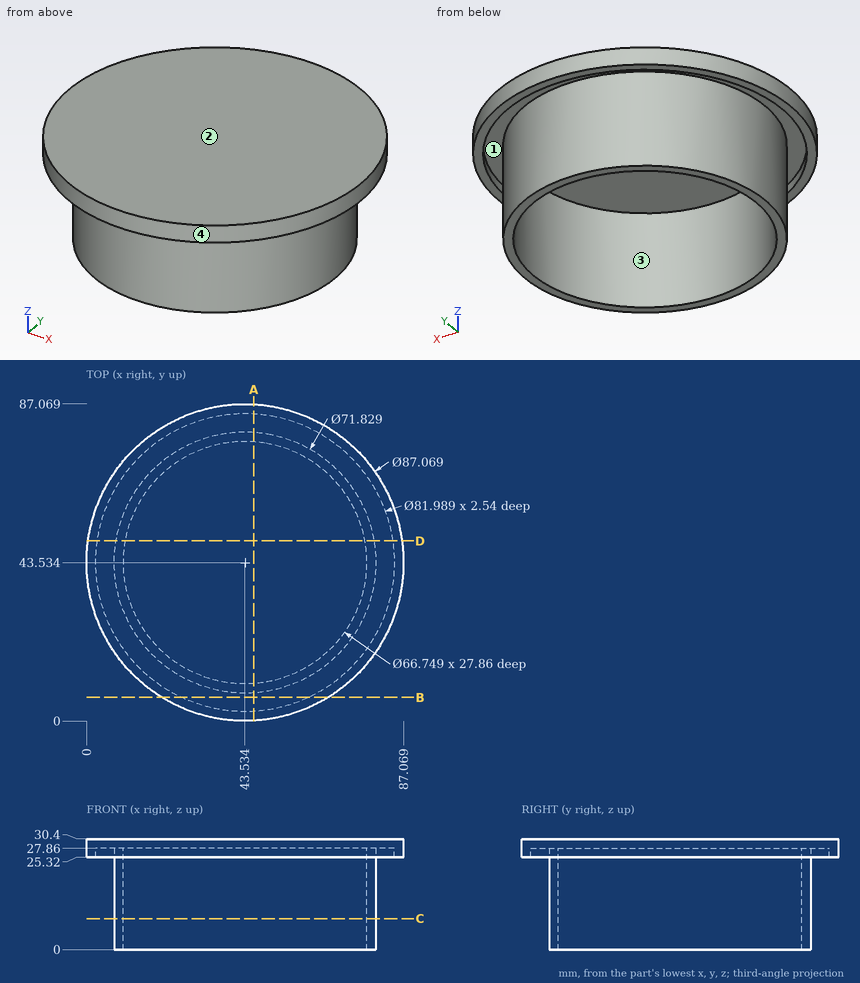
Source: three-view drawing plus pictorial views. Frame: mm from the lowest corner of the part. Coordinates: 2 decimals unless noted, no trailing zeros. Loops run counter-clockwise (first coordinate to the right, second up) from the corner with the lowest first, then second, coordinate; pieces in that order, holes last. Notation, with made-up numbers: (-26.75, 81) - (12.25, 81) arc R34 ccw to (12.25, 112) - close; hole circle Ø1 at (72, -22.75). An arc over 180 degrees is marked (long way). Answer in a Markdown table with one row per item. Add a question column.
Item 1: Contact query for flat-ended pins moving along their axis: P1, Ø1, axis at x = 64, z = 15.5, coming from the -Y side; P2, Ø6, axis at x = 51, y = 46.5, coming from the -Z side; P3, Ø1.5, axis at y = 56, z = 17, coming from the +X side (1 decimal). Output: stop coordinate, or through.
Item 2: Section query B-B on y = 6.5. Return the cut outline in (x, z), then the cut area to 3 significant figures.
Item 3: Section query C-C on z = 8.5. Return the cut outline in (x, y) (1 decimal).
Item 4: Section query A-A on x = 46. Return the cut outline in (y, z) (1 decimal).
Item 5: Mould query, pull axis X, two halves, no side actions, for the marked faces 1, 2, 3 and 4. Classes: released by +X, released by -X, zero draft, split by the parting line, or undercut.
Item 6: Line query: line 1 along Z through (x, y) = (21.5, 57.5); line 2 along X through (y, z) = (21, 24) (1 decimal); line 3 along Y through (x, z) = (32, 6.5) (1 decimal). Output: solid intervals per line, ascending. Write a range as [from, to].
Item 7: Section query D-D on y = 49.5. Return the cut outline in (x, z).
Recorded:
| question | item | result |
|---|---|---|
| 1 | P1 | y = 13.68 |
| 1 | P2 | z = 27.86 |
| 1 | P3 | x = 77.5 |
| 2 | outline | (20.65, 25.32) - (25.96, 25.32) - (25.96, 27.86) - (61.11, 27.86) - (61.11, 25.32) - (66.42, 25.32) - (66.42, 30.4) - (20.65, 30.4) - close |
| 2 | area | 143 mm^2 |
| 3 | outline | circle Ø71.8 at (43.5, 43.5); hole circle Ø66.7 at (43.5, 43.5) |
| 4 | outline | (0.1, 25.3) - (2.6, 25.3) - (2.6, 27.9) - (7.7, 27.9) - (7.7, 0) - (10.3, 0) - (10.3, 27.9) - (76.8, 27.9) - (76.8, 0) - (79.4, 0) - (79.4, 27.9) - (84.5, 27.9) - (84.5, 25.3) - (87, 25.3) - (87, 30.4) - (0.1, 30.4) - close |
| 5 | face 1 | undercut |
| 5 | face 2 | zero draft |
| 5 | face 3 | undercut |
| 5 | face 4 | split by the parting line |
| 6 | line 1 | [27.86, 30.4] |
| 6 | line 2 | [15.6, 18.9], [68.2, 71.5] |
| 6 | line 3 | [9.5, 12.2], [74.9, 77.5] |
| 7 | outline | (0.41, 25.32) - (2.98, 25.32) - (2.98, 27.86) - (8.12, 27.86) - (8.12, 0) - (10.7, 0) - (10.7, 27.86) - (76.37, 27.86) - (76.37, 0) - (78.95, 0) - (78.95, 27.86) - (84.09, 27.86) - (84.09, 25.32) - (86.66, 25.32) - (86.66, 30.4) - (0.41, 30.4) - close |
